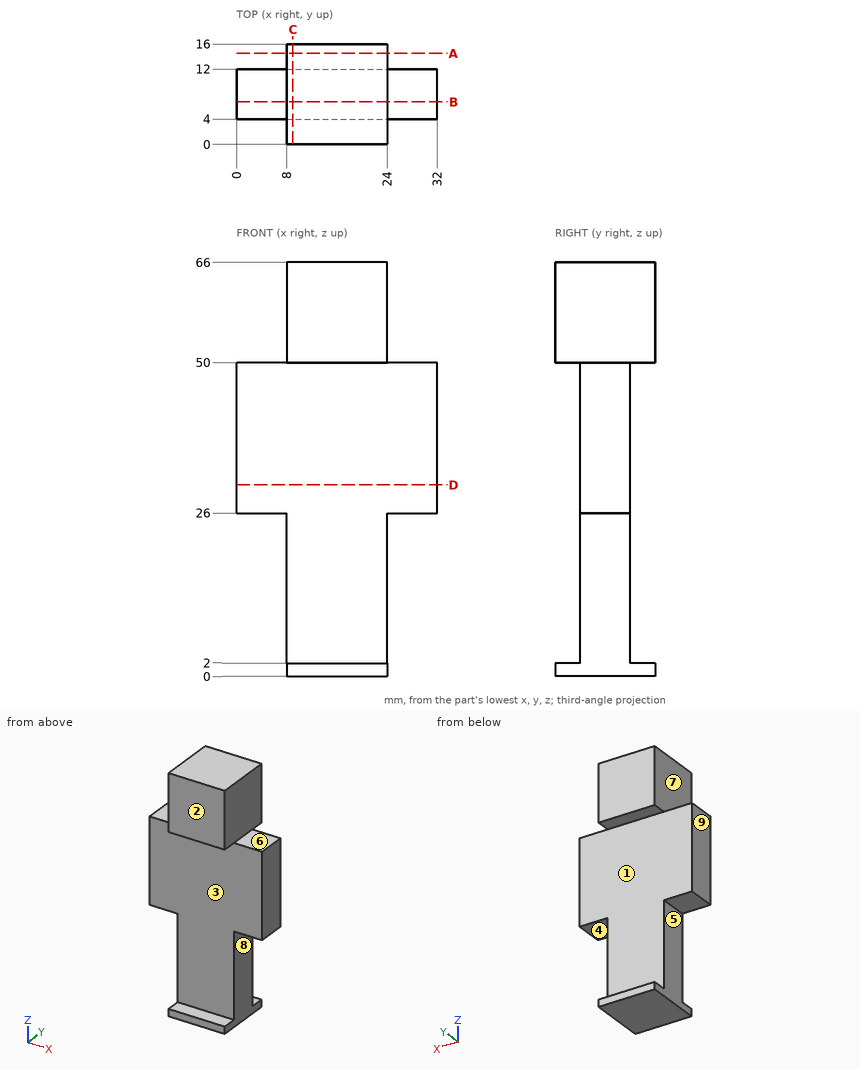
Answer from the drawing. Dimensions are ordinates in mm from the lowest x, y and z of the part. A direction names the side the tool comes from. Coordinates: 2 decimals unless noted, no trailing zeros. Order: outer loops, then holes, each group sorted by start corner. A loop starts at its lowest first (then second) coordinate and runs counter-clockwise, first axis right, second up. Notation, with made-up numbers: (-25, 50) - (-8, 50) arc R33 cw to (-8, 81) - close; hole circle Ø1 at (-9, -5). An arc over 180 degrees is marked (long way). Put each result on its own line as item: value. Start each with the question number.
1) For the marked faces 5, 6, 7, 8 and 9, determine the directions among +Z, -Z, +X, -X, +Y, -Y from which every point of the face is accessible in a straight line to the end or side of a thin tool.
2) Find section C-C (x = 9). Give the vertices of the cut face in (y, z), plus the area to 3 significant figures.
3) Find the intervals of material crossed by line 1 (Z direction, x = 12, y = 13.5); line 2 (X direction, y = 14, z = 58.5); line 3 (Y direction, x = 22, z = 13), in increasing order. Write a range as from..to.
4) For a pull along Z with two mould halves and no side action, classify the marked faces 1, 2, 3 and 4 as released by +Z, released by -Z, zero draft, split by the parting line, or undercut.
5) Find section D-D (z = 30.5). Give the vertices of the cut face in (x, y), plus the area to 3 significant figures.
6) Flat-ended cylindrical pins translate along their axes: pin 1 (6.5 mm diameter, centred on x = 27.5, y = 6.5, fed in from +Z); pin 2 (6.5 mm diameter, centred on x = 27.5, y = 6, fed in from -Z); pin 3 (1.5 mm diameter, centred on x = 15.5, z = 15, fed in from +Y). Find the tip coordinate at first contact, or state that the pin passes through.
7) Find section A-A (y = 14.5). Give the vertices of the cut face in (x, z), plus the area to 3 significant figures.
8) Find section B-B (y = 6.75). Give the vertices of the cut face in (x, z).
Results list:
1. face 5: -Z, -X, +Y, -Y
1. face 6: +Z, +X, +Y, -Y
1. face 7: +Z, -X, +Y, -Y
1. face 8: -Z, +X, +Y, -Y
1. face 9: +Z, -Z, -X, +Y, -Y
2. outline: (0, 0) - (16, 0) - (16, 2) - (12, 2) - (12, 50) - (16, 50) - (16, 66) - (0, 66) - (0, 50) - (4, 50) - (4, 2) - (0, 2) - close
2. area: 672 mm^2
3. line 1: z = 0..2, 50..66
3. line 2: x = 8..24
3. line 3: y = 4..12
4. face 1: undercut
4. face 2: zero draft
4. face 3: undercut
4. face 4: released by -Z
5. outline: (0, 4) - (32, 4) - (32, 12) - (0, 12) - close
5. area: 256 mm^2
6. pin 1: stops at z = 50
6. pin 2: stops at z = 26
6. pin 3: stops at y = 12
7. outline: (8, 0) - (24, 0) - (24, 2) - (8, 2) - close; (8, 50) - (24, 50) - (24, 66) - (8, 66) - close
7. area: 288 mm^2
8. outline: (0, 26) - (8, 26) - (8, 0) - (24, 0) - (24, 26) - (32, 26) - (32, 50) - (24, 50) - (24, 66) - (8, 66) - (8, 50) - (0, 50) - close
